Input: part model. Units: mm. Frame: model coordinates. Face numbers are marked on the shaded views. A direction names the side the tool comes from. Round coordinates to 2 decimals unless told otherwise and drop trailing zeros. Order: outer loops, then holes, each group sorted by start corner. A loop starts at its lowest first (then second) coordinate and runs counter-clockwise, first axis right, second up.
Item 1: Line query: L1, parallel to Z at x = 7, y = 12; L2, parallel to X at y = 10.5, z = 15; L3, parallel to Z at x = -1, y = 12. Output: solid intervals per line, ascending.
Item 2: Reachability of the marked faces 4, 5 and 6 from +Z, -Z, +X, -X, +Y, -Y: full face, straight path, thin tool, end or side. Return the list, or none.
Item 3: Mould query, pull axis Z, two halves, no side actions, for the marked faces 1, 2 and 3. Classes: released by +Z, released by -Z, zero draft, split by the parting line, or undercut.
Item 4: Cut plane B-B on y = 11.5. Give the number of separate pieces and of enclosed holes in the cut face, then the cut area to 3 significant figures.
Item 5: Cut plane A-A on z = 6.75. Output: boundary loops of the cut face in (x, y).
Item 6: First-contact query: pin 1 (4.5 mm diameter, centred on x = 0, z = -13.5, fed in from -Y); pin 2 (2.5 mm diameter, centred on y = 11.5, z = 0, fed in from -X); pin 3 (4 mm diameter, centred on y = 5, z = -8.5, fed in from -X); pin 4 (1.5 mm diameter, centred on y = 5, z = 5.5, fed in from +X). Flat tips, straight axial feed; report the tip coordinate or a pass-through.
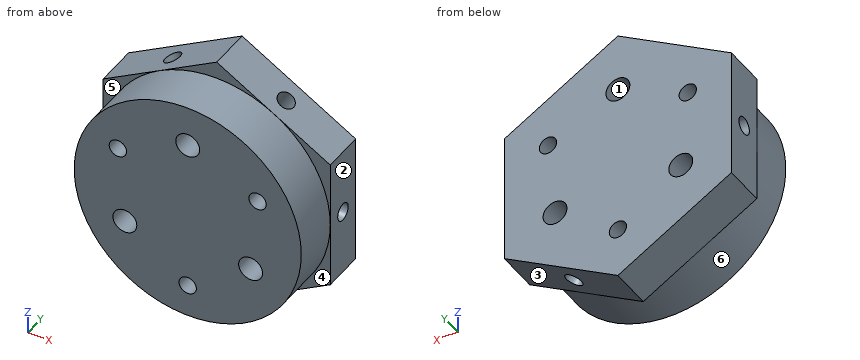
```python
from build123d import *

# Parameters (mm, degrees)
SKETCH_1_R          = 19
SKETCH_1_R_2        = 1.45
SKETCH_1_R_3        = 2
EXTRUDE_1_DEPTH     = 15
SKETCH_2_R          = 1.45
SKETCH_2_R_2        = 2
EXTRUDE_2_DEPTH     = 7
SKETCH_3_R          = 1.45
CUT_EXTRUDE_1_DEPTH = 8
SKETCH_4_R          = 1.45
CUT_EXTRUDE_2_DEPTH = 8
SKETCH_5_R          = 1.45
CUT_EXTRUDE_3_DEPTH = 8
SKETCH_6_R          = 1.45
CUT_EXTRUDE_4_DEPTH = 8
SKETCH_7_R          = 1.45
CUT_EXTRUDE_5_DEPTH = 8


with BuildPart() as part:
    # 草图1 → 凸台-拉伸1 (new body)
    with BuildSketch(Plane(origin=(0, 0, 0), x_dir=(1, 0, 0), z_dir=(0, 1, 0))):
        Circle(SKETCH_1_R)
        with Locations((0, 13.5)):
            Circle(SKETCH_1_R_2, mode=Mode.SUBTRACT)
        with Locations((-11.691342951, -6.75)):
            Circle(SKETCH_1_R_2, mode=Mode.SUBTRACT)
        with Locations((11.691342951, -6.75)):
            Circle(SKETCH_1_R_2, mode=Mode.SUBTRACT)
        with Locations((-10.522208656, 6.075)):
            Circle(SKETCH_1_R_3, mode=Mode.SUBTRACT)
        with Locations((0, -12.15)):
            Circle(SKETCH_1_R_3, mode=Mode.SUBTRACT)
        with Locations((10.522208656, 6.075)):
            Circle(SKETCH_1_R_3, mode=Mode.SUBTRACT)
    extrude(amount=EXTRUDE_1_DEPTH)

    # 草图2 → 凸台-拉伸2 (add)
    with BuildSketch(Plane(origin=(0, 15, 0), x_dir=(1, 0, 0), z_dir=(0, 1, 0))):
        Polygon((0, 21.939310229), (-19, 10.969655115), (-19, -10.969655115), (0, -21.939310229), (19, -10.969655115), (19, 10.969655115), align=None)
        with Locations((0, 13.5)):
            Circle(SKETCH_2_R, mode=Mode.SUBTRACT)
        with Locations((-10.522208656, 6.075)):
            Circle(SKETCH_2_R_2, mode=Mode.SUBTRACT)
        with Locations((10.522208656, 6.075)):
            Circle(SKETCH_2_R_2, mode=Mode.SUBTRACT)
        with Locations((-11.691342951, -6.75)):
            Circle(SKETCH_2_R, mode=Mode.SUBTRACT)
        with Locations((0, -12.15)):
            Circle(SKETCH_2_R_2, mode=Mode.SUBTRACT)
        with Locations((11.691342951, -6.75)):
            Circle(SKETCH_2_R, mode=Mode.SUBTRACT)
    extrude(amount=-EXTRUDE_2_DEPTH)

    # 草图3 → 切除-拉伸1 (cut)
    with BuildSketch(Plane(origin=(9.5, 0, 16.454482672), x_dir=(0.866025404, 0, -0.5), z_dir=(0.5, 0, 0.866025404))):
        with Locations((0, 11.5)):
            Circle(SKETCH_3_R)
    extrude(amount=-CUT_EXTRUDE_1_DEPTH, mode=Mode.SUBTRACT)

    # 草图4 → 切除-拉伸2 (cut)
    with BuildSketch(Plane(origin=(-9.5, 0, 16.454482672), x_dir=(0.866025404, 0, 0.5), z_dir=(-0.5, 0, 0.866025404))):
        with Locations((0, 11.5)):
            Circle(SKETCH_4_R)
    extrude(amount=-CUT_EXTRUDE_2_DEPTH, mode=Mode.SUBTRACT)

    # 草图5 → 切除-拉伸3 (cut)
    with BuildSketch(Plane.ZY.offset(19)):
        with Locations((0, 11.5)):
            Circle(SKETCH_5_R)
    extrude(amount=-CUT_EXTRUDE_3_DEPTH, mode=Mode.SUBTRACT)

    # 草图6 → 切除-拉伸4 (cut)
    with BuildSketch(Plane(origin=(19, 0, 0), x_dir=(0, 0, -1), z_dir=(1, 0, 0))):
        with Locations((0, 11.5)):
            Circle(SKETCH_6_R)
    extrude(amount=-CUT_EXTRUDE_4_DEPTH, mode=Mode.SUBTRACT)

    # 草图7 → 切除-拉伸5 (cut)
    with BuildSketch(Plane(origin=(9.5, 0, -16.454482672), x_dir=(-0.866025404, 0, -0.5), z_dir=(0.5, 0, -0.866025404))):
        with Locations((0, 11.5)):
            Circle(SKETCH_7_R)
    extrude(amount=-CUT_EXTRUDE_5_DEPTH, mode=Mode.SUBTRACT)


solid = part.part
```
From the geometry:
1. L1: z = -17.9 to -14.85, -9.4 to 9.4, 14.85 to 17.9
1. L2: x = -12.02 to -9.87, -7.45 to 7.45, 9.87 to 12.02
1. L3: z = -21.36 to -14.55, -12.45 to 10.42, 13.88 to 21.36
2. face 4: -Z, +X, -Y
2. face 5: +Z, -X, -Y
2. face 6: -Y
3. face 1: undercut
3. face 2: zero draft
3. face 3: released by -Z
4. separate pieces: 1
4. enclosed holes: 6
4. area: 1,080 mm2
5. outline: (-19, 8) - (-17.76, 8) - (-17.76, 0) - (-13.14, 0) - (-13.14, 15) - (-19, 15) - close; (-10.24, 0) - (10.24, 0) - (10.24, 15) - (-10.24, 15) - close; (13.14, 0) - (17.76, 0) - (17.76, 8) - (19, 8) - (19, 15) - (13.14, 15) - close
6. pin 1: stops at y = 0
6. pin 2: stops at x = -11
6. pin 3: stops at x = -17.85
6. pin 4: stops at x = 18.4
